Geometry check sheet. Reference: the model listing, model coordinates, mm. A direction names the side the tool comes from. Coordinates: 2 decimals unless noted, no trailing zeros. Loops run counter-clockwise (first coordinate to the right, second up) from the corner with the lowest first, then second, coordinate; pieces in that order, holes last.
from build123d import *

# Parameters (mm, degrees)
SKETCH012_W     = 66
SKETCH012_H     = 98
PAD006_DEPTH    = 15
SKETCH013_W     = 60
SKETCH013_H     = 92
POCKET008_DEPTH = 6.5
FILLET008_R     = 3
SKETCH014_W     = 59
SKETCH014_H     = 84
POCKET009_DEPTH = 6.5
POCKET010_DEPTH = 7
FILLET009_R     = 6
CHAMFER005_SIZE = 1.6
CHAMFER006_SIZE = 2


with BuildPart() as part:
    # Sketch012 → Pad006 (new body)
    with BuildSketch(Plane.XY):
        Rectangle(SKETCH012_W, SKETCH012_H)
    extrude(amount=PAD006_DEPTH)

    # Sketch013 (on Face6 of Pad006) → Pocket008 (cut)
    with BuildSketch(Plane.XY.offset(15)):
        Rectangle(SKETCH013_W, SKETCH013_H)
    extrude(amount=-POCKET008_DEPTH, mode=Mode.SUBTRACT)

    # Fillet008
    fillet008_edges = [part.edges().sort_by_distance(p)[0] for p in [
        (30, 46, 11.75),
        (-30, 46, 11.75),
        (-30, -46, 11.75),
        (30, -46, 11.75),
    ]]
    fillet(fillet008_edges, radius=FILLET008_R)

    # Sketch014 (on Face11 of Pocket008) → Pocket009 (cut)
    with BuildSketch(Plane.XY.offset(8.5)):
        Rectangle(SKETCH014_W, SKETCH014_H)
    extrude(amount=-POCKET009_DEPTH, mode=Mode.SUBTRACT)

    # Sketch015 (on Face13 of Pocket009) → Pocket010 (cut)
    with BuildSketch(Plane.XZ.offset(49)):
        with BuildLine():
            ThreePointArc((-18.9, 8.5), (-22.05, 5.35), (-18.9, 2.2))
            Line((-18.9, 2.2), (-12.6, 2.2))
            ThreePointArc((-12.6, 2.2), (-9.45, 5.35), (-12.6, 8.5))
            Line((-12.6, 8.5), (-18.9, 8.5))
        make_face()
    extrude(amount=-POCKET010_DEPTH, mode=Mode.SUBTRACT)

    # Fillet009
    fillet009_edges = [part.edges().sort_by_distance(p)[0] for p in [
        (33, -49, 7.5),
        (33, 49, 7.5),
        (-33, -49, 7.5),
        (-33, 49, 7.5),
    ]]
    fillet(fillet009_edges, radius=FILLET009_R)

    # Chamfer005
    chamfer005_edges = [part.edges().sort_by_distance(p)[0] for p in [
        (0, 49, 0),
        (-31.242641, 47.242641, 0),
        (31.242641, 47.242641, 0),
        (-33, 0, 0),
        (33, 0, 0),
        (-31.242641, -47.242641, 0),
        (31.242641, -47.242641, 0),
        (0, -49, 0),
    ]]
    chamfer(chamfer005_edges, length=CHAMFER005_SIZE)

    # Chamfer006
    chamfer006_edges = [part.edges().sort_by_distance(p)[0] for p in [
        (-33, 0, 15),
    ]]
    chamfer(chamfer006_edges, length=CHAMFER006_SIZE)


solid = part.part
(1) Sectioned sample at D-D on z = 5.35. Record the cut outline in (x, y), and give its area (3 significant figures).
Findings:
outline: (-33, -43) arc R6 ccw to (-27, -49) - (-22.05, -49) - (-22.05, -42) - (-29.5, -42) - (-29.5, 42) - (29.5, 42) - (29.5, -42) - (-9.45, -42) - (-9.45, -49) - (27, -49) arc R6 ccw to (33, -43) - (33, 43) arc R6 ccw to (27, 49) - (-27, 49) arc R6 ccw to (-33, 43) - close
area: 1,390 mm2
(2) Sectioned sample at B-B on z = 11.5. Record the cut outline in (x, y), and give its area (3 significant figures).
Findings:
outline: (-33, -43) arc R6 ccw to (-27, -49) - (27, -49) arc R6 ccw to (33, -43) - (33, 43) arc R6 ccw to (27, 49) - (-27, 49) arc R6 ccw to (-33, 43) - close; hole (-30, -43) arc R3 ccw to (-27, -46) - (27, -46) arc R3 ccw to (30, -43) - (30, 43) arc R3 ccw to (27, 46) - (-27, 46) arc R3 ccw to (-30, 43) - close
area: 925 mm2
(3) Sectioned sample at A-A on x = -16. Record the cut outline in (y, z), and give its area (3 significant figures).
Findings:
outline: (-49, 1.6) - (-47.4, 0) - (47.4, 0) - (49, 1.6) - (49, 13) - (47, 15) - (46, 15) - (46, 8.5) - (42, 8.5) - (42, 2) - (-42, 2) - (-42, 2.2) - (-49, 2.2) - close; (-49, 8.5) - (-46, 8.5) - (-46, 15) - (-47, 15) - (-49, 13) - close
area: 275 mm2
(4) Draft check along Y on faces 1 (the cylindrical face through (-9.45, -45.55, 5.28)), 2 (the conical face through (-30.504, -46.582, 0.611)), 3 (the cylindrical face through (29.1, -45.14, 11.7)). Enter one of: +Y half, -Y half, draft (parallel to the pull), parting line (faces both ways), or undercut.
Findings:
face 1: draft
face 2: -Y half
face 3: undercut
(5) Sectioned sample at C-C on y = 16. Record the cut outline in (x, z), and give its area (3 significant figures).
Findings:
outline: (-33, 1.6) - (-31.4, 0) - (31.4, 0) - (33, 1.6) - (33, 13) - (31, 15) - (30, 15) - (30, 8.5) - (29.5, 8.5) - (29.5, 2) - (-29.5, 2) - (-29.5, 8.5) - (-30, 8.5) - (-30, 15) - (-31, 15) - (-33, 13) - close
area: 210 mm2
(6) Access from +Z, -Z, +X, -X, +Y, -Y to the whole of each face (thin tool, end or side, straight path). Record for faces 4 (the flat face through (-16, -46, 2.2)), 5 (the cylindrical face through (29.14, 45.1, 11.7)), 6 (the conical face through (30.504, 46.582, 0.611)).
Findings:
face 4: -Y
face 5: +Z
face 6: -Z, +X, +Y
(7) Scan lines: L1, parallel to X at y = 8.5, z = 10; L2, parallel to Y at x = -26, z = 4; L3, parallel to X at y = -17, z = 7.25. Record each from-to range of solid material in increasing order.
Findings:
L1: x = -33 to -30, 30 to 33
L2: y = -49 to -42, 42 to 49
L3: x = -33 to -29.5, 29.5 to 33
(8) Gauge pin test, flat end, axial feed: pin 1 Ø17.5 at (x, y) = (6.5, -17.5) entering from +Z. Record the tip position at first contact, or that the pin passes through.
Findings:
pin 1: stops at z = 2
